Source: three-view drawing plus pictorial views. Frame: mm from the lowest corner of the part. A direction names the side the tool comes from. Round coordinates to 2 decimals unless told otherwise and drop trailing zeros. Loops run counter-clockwise (first coordinate to the right, second up) from the corner with the lowest first, then second, coordinate; pieces in that order, holes last. Notation, with made-up numbers: (-4.5, 22) -> (30.5, 22) arc R13 ccw to (30.5, 29) -> close; hole circle Ø3 at (79, 2). An arc over 180 degrees is marked (long way). One line per question, with ' | ' between items. Start each with the question number.
Q1. Access query for the marked faces 4, 5, 6, 7 and 8. Directions: +Z, -Z, +X, -X, +Y, -Y. A direction counts if a zero-diameter tool reaches every point of the face in a straight line with its end or side. Return the directions, or none.
Q2. Cut plane C-C on x = 57. Return loops of the section in (y, z) (1 decimal), and give its area (3 significant figures).
Q3. Cut plane A-A on x = 5. Return loops of the section in (y, z), and give its area (3 significant figures).
Q4. Material intervals for L1, parallel to X at y = 34.5, z = 34; L2, parallel to X at y = 25.5, z = 72.5; L3, parallel to X at y = 15.5, z = 94, sorted ascending.
Q5. Mould query, pull axis Z, two halves, no side actions, for the marked faces 1, 2 and 3. Classes: pulls with the +Z half, pulls with the -Z half, needs draft (parallel to the pull), parting line crosses it, or undercut.
Q6. Cut plane B-B on y = 4. Return loops of the section in (x, z).
Q7. Cut plane D-D on x = 82. Return loops of the section in (y, z) (1 decimal), and give its area (3 significant figures).
Q8. Contact query for flat-ended pins moving along their axis: P1, Ø3.5, axis at y = 19, z = 95.5, coming from the +X side; P2, Ø7.5, axis at y = 18, z = 98, coming from the -X side; P3, Ø12, axis at y = 25, z = 83, coming from the +X side. Output: stop coordinate, or through.
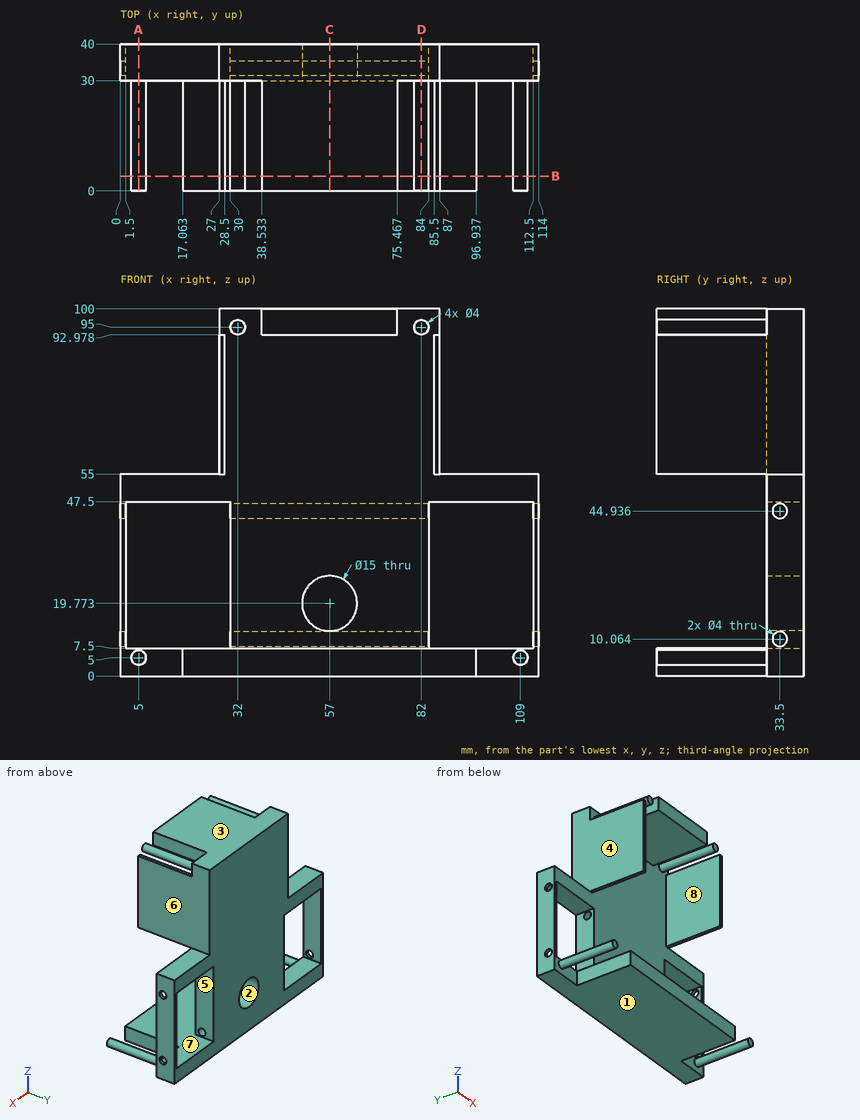
Results:
1) face 4: +Z, -X, +Y, -Y | face 5: +Y, -Y | face 6: +Z, +X, +Y, -Y | face 7: -Y | face 8: +Z, -Y
2) outline: (0, 0) -> (40, 0) -> (40, 12.3) -> (30, 12.3) -> (30, 7.5) -> (0, 7.5) -> close; (0, 93) -> (30, 93) -> (30, 27.3) -> (40, 27.3) -> (40, 100) -> (0, 100) -> close; hole circle Ø4 at (33.5, 10.1); hole circle Ø4 at (33.5, 44.9) | area: 1,260 mm^2
3) outline: (0, 3) -> (30, 3) -> (30, 0) -> (40, 0) -> (40, 7.5) -> (30, 7.5) -> (30, 7) -> (0, 7) -> close; (30, 47.5) -> (40, 47.5) -> (40, 55) -> (30, 55) -> close | area: 270 mm^2
4) L1: 0 to 1.5, 30 to 84, 112.5 to 114 | L2: 27 to 28.5, 85.5 to 87 | L3: 30.27 to 33.73, 38.53 to 75.47, 80.27 to 83.73
5) face 1: pulls with the -Z half | face 2: undercut | face 3: pulls with the +Z half
6) outline: circle Ø4 at (5, 5); (17.06, 0) -> (96.94, 0) -> (96.94, 7.5) -> (17.06, 7.5) -> close; (27, 55) -> (28.5, 55) -> (28.5, 92.98) -> (27, 92.98) -> close; circle Ø4 at (32, 95); (38.53, 92.98) -> (75.47, 92.98) -> (75.47, 100) -> (38.53, 100) -> close; circle Ø4 at (82, 95); (85.5, 55) -> (87, 55) -> (87, 92.98) -> (85.5, 92.98) -> close; circle Ø4 at (109, 5)
7) outline: (0, 0) -> (40, 0) -> (40, 100) -> (30, 100) -> (30, 97) -> (0, 97) -> (0, 93) -> (30, 93) -> (30, 7.5) -> (0, 7.5) -> close; hole circle Ø4 at (33.5, 10.1); hole circle Ø4 at (33.5, 44.9) | area: 1,320 mm^2
8) P1: x = 84 | P2: x = 30 | P3: x = 87
